from build123d import *

# Parameters (mm, degrees)
F0_W     = 100
F0_H     = 100
F1_DEPTH = 20
F2_R     = 16.5
F3_DEPTH = 15
F4_T     = -2.5


with BuildPart() as f1:
    # F0 (on Top) → F1 (new body)
    with BuildSketch(Plane.XY):
        with Locations((26.9842460752, 19.6610757008)):
            Rectangle(F0_W, F0_H)
    extrude(amount=F1_DEPTH)

    # F2 (on face) → F3 (cut)
    with BuildSketch(Plane.XY.offset(20)):
        with Locations((1.9842460752, 44.6610757008)):
            Circle(F2_R)
        with Locations((51.9842460752, 44.6610757008)):
            Circle(F2_R)
        with Locations((51.9842460752, -5.3389242992)):
            Circle(F2_R)
        with Locations((1.9842460752, -5.3389242992)):
            Circle(F2_R)
    extrude(amount=-F3_DEPTH, mode=Mode.SUBTRACT)

    # F4
    f4_openings = [f1.faces().sort_by_distance(p)[0] for p in [
        (26.984246, 19.661076, 0),
    ]]
    offset(amount=F4_T, openings=f4_openings, kind=Kind.INTERSECTION)


solid = f1.part
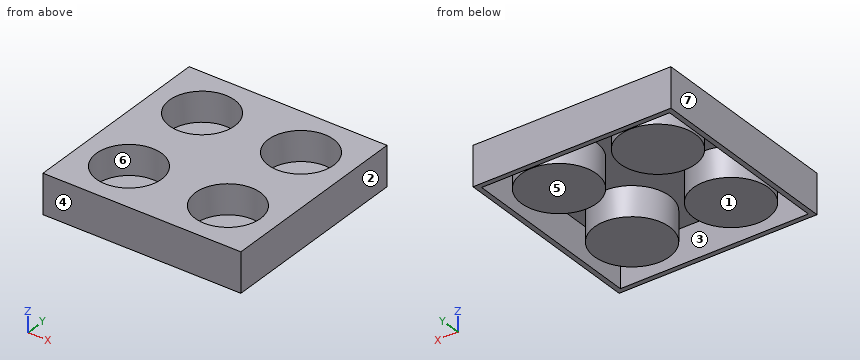
Can you work these out from the model? Positions are in its coordinate system, mm. Face numbers are marked on the shaded views. A direction names the side the tool comes from. Coordinates: 2 decimals unless noted, no trailing zeros. Write each loop counter-clockwise with the first axis right and the second up, starting at its lowest first coordinate (ties: lowest second). Pieces come first, ordered by that corner, then holes.
Q1. For P1, Ø10, axis at x = -3, y = 46.5, coming from the +Z side, with a flat end and sliding along its axis, tell me the tip position at first contact or that it passes through.
Results found:
P1: stops at z = 5
Q2. Please list where these lines run through material, in increasing order: L1, parallel to Y at x = 1, z = 4; L2, parallel to X at y = -1, z = 14.5; L3, parallel to X at y = -3, z = 7.75.
Results found:
L1: y = -30.34 to -27.84, -24.31 to 13.64, 25.69 to 63.64, 67.16 to 69.66
L2: x = -23.02 to -20.52, -16.51 to -13.94, 17.9 to 20.48, 33.49 to 36.06, 67.9 to 70.48, 74.48 to 76.98
L3: x = -23.02 to -20.52, -16.87 to -14.35, 18.32 to 20.84, 33.13 to 35.65, 68.32 to 70.84, 74.48 to 76.98
Q3. Imagine slicing it at B-B, the plane x = 22.5. List the corners of the cut face in (y, z) for me, plus the area to 4 significant figures.
Results found:
outline: (-30.34, 0) - (-27.84, 0) - (-27.84, 17.5) - (67.16, 17.5) - (67.16, 0) - (69.66, 0) - (69.66, 20) - (-30.34, 20) - close
area: 337.5 mm2
Q4. If we mould it in two halves opening along Y, with no side actions, what happens to the marked faces 1, 2, 3 and 4? For each: +Y half, -Y half, draft (parallel to the pull), parting line (faces both ways), or undercut.
Results found:
face 1: undercut
face 2: draft
face 3: undercut
face 4: -Y half
Q5. Which directions (+Z, -Z, +X, -X, +Y, -Y) give clear straight access to the entire face, cutting with the end or side of a thin tool? Please do the marked faces 5, 6 and 7.
Results found:
face 5: -Z
face 6: +Z
face 7: +Z, -Z, -X, +Y, -Y
Q6. Imagine slicing it at D-D, the plane y = -1.5. List the corners of the cut face in (x, z) for me.
Results found:
outline: (-23.02, 0) - (-20.52, 0) - (-20.52, 17.5) - (-16.62, 17.5) - (-16.62, 2.5) - (20.59, 2.5) - (20.59, 17.5) - (33.38, 17.5) - (33.38, 2.5) - (70.59, 2.5) - (70.59, 17.5) - (74.48, 17.5) - (74.48, 0) - (76.98, 0) - (76.98, 20) - (68.03, 20) - (68.03, 5) - (35.94, 5) - (35.94, 20) - (18.03, 20) - (18.03, 5) - (-14.06, 5) - (-14.06, 20) - (-23.02, 20) - close
Q7. Imagine slicing it at A-A, the plane z = 9. Count the separate pieces of the cut face and the enclosed holes in it, plus the area to 3 significant figures.
Results found:
separate pieces: 5
enclosed holes: 5
area: 2,090 mm2
Q8. Imagine slicing it at C-C, the plane y = 38.5. List the corners of the cut face in (x, z) for me.
Results found:
outline: (-23.02, 0) - (-20.52, 0) - (-20.52, 17.5) - (-15.99, 17.5) - (-15.99, 2.5) - (19.96, 2.5) - (19.96, 17.5) - (34.01, 17.5) - (34.01, 2.5) - (69.96, 2.5) - (69.96, 17.5) - (74.48, 17.5) - (74.48, 0) - (76.98, 0) - (76.98, 20) - (67.29, 20) - (67.29, 5) - (36.68, 5) - (36.68, 20) - (17.29, 20) - (17.29, 5) - (-13.32, 5) - (-13.32, 20) - (-23.02, 20) - close
